```python
from build123d import *

# Parameters (mm, degrees)
BOSS_EXTRUDE1_DEPTH = 50
SHELL1_T            = -1.5
SKETCH2_R           = 2.5
CUT_EXTRUDE1_DEPTH  = 50
SKETCH3_OUTSIDE_W   = 189.504
SKETCH3_OUTSIDE_H   = 139.504
CUT_EXTRUDE2_DEPTH  = 5
CUT_EXTRUDE2_TAPER  = 0.5
FILLET1_R           = 0.5
CHAMFER1_SIZE       = 1.25


with BuildPart() as part:
    # Sketch1 → Boss-Extrude1 (new body)
    with BuildSketch(Plane(origin=(0, 0, 0), x_dir=(1, 0, 0), z_dir=(0, 1, 0))):
        with BuildLine():
            Line((-72.5, -50), (72.5, -50))
            ThreePointArc((72.5, -50), (74.267766953, -49.267766953), (75, -47.5))
            Line((75, -47.5), (75, 47.5))
            ThreePointArc((75, 47.5), (74.267766953, 49.267766953), (72.5, 50))
            Line((72.5, 50), (-72.5, 50))
            ThreePointArc((-72.5, 50), (-74.267766953, 49.267766953), (-75, 47.5))
            Line((-75, 47.5), (-75, -47.5))
            ThreePointArc((-75, -47.5), (-74.267766953, -49.267766953), (-72.5, -50))
        make_face()
    extrude(amount=BOSS_EXTRUDE1_DEPTH)

    # Shell1
    shell1_openings = [part.faces().sort_by_distance(p)[0] for p in [
        (0, 50, 0),
    ]]
    offset(amount=SHELL1_T, openings=shell1_openings, kind=Kind.INTERSECTION)

    # Sketch2 → Cut-Extrude1 (cut)
    with BuildSketch(Plane(origin=(0, 1.5, 0), x_dir=(1, 0, 0), z_dir=(0, 1, 0))):
        with Locations((-65, 40)):
            Circle(SKETCH2_R)
        with Locations((65, 40)):
            Circle(SKETCH2_R)
        with Locations((65, -40)):
            Circle(SKETCH2_R)
        with Locations((-65, -40)):
            Circle(SKETCH2_R)
    extrude(amount=-CUT_EXTRUDE1_DEPTH, mode=Mode.SUBTRACT)

    # Sketch3 outside → Cut-Extrude2 (cut)
    with BuildSketch(Plane(origin=(0, 50, 0), x_dir=(1, 0, 0), z_dir=(0, 1, 0))):
        Rectangle(SKETCH3_OUTSIDE_W, SKETCH3_OUTSIDE_H)
        with BuildLine():
            Line((-69.232233047, -45.732233047), (69.232233047, -45.732233047))
            ThreePointArc((69.232233047, -45.732233047), (70.292893219, -45.292893219), (70.732233047, -44.232233047))
            Line((70.732233047, -44.232233047), (70.732233047, 44.232233047))
            ThreePointArc((70.732233047, 44.232233047), (70.292893219, 45.292893219), (69.232233047, 45.732233047))
            Line((69.232233047, 45.732233047), (-69.232233047, 45.732233047))
            ThreePointArc((-69.232233047, 45.732233047), (-70.292893219, 45.292893219), (-70.732233047, 44.232233047))
            Line((-70.732233047, 44.232233047), (-70.732233047, -44.232233047))
            ThreePointArc((-70.732233047, -44.232233047), (-70.292893219, -45.292893219), (-69.232233047, -45.732233047))
        make_face(mode=Mode.SUBTRACT)
    extrude(amount=-CUT_EXTRUDE2_DEPTH, taper=CUT_EXTRUDE2_TAPER, mode=Mode.SUBTRACT)

    # Fillet1
    fillet1_edges = [part.edges().sort_by_distance(p)[0] for p in [
        (-75, 0, 0),
        (-74.267766953, 0, -49.267766953),
        (0, 0, -50),
        (74.267766953, 0, -49.267766953),
        (75, 0, 0),
        (74.267766953, 0, 49.267766953),
        (0, 0, 50),
        (-74.267766953, 0, 49.267766953),
    ]]
    fillet(fillet1_edges, radius=FILLET1_R)

    # Chamfer1
    chamfer1_edges = [part.edges().sort_by_distance(p)[0] for p in [
        (-67.5, 1.5, -40),
        (62.5, 1.5, -40),
        (62.5, 1.5, 40),
        (-67.5, 1.5, 40),
    ]]
    chamfer(chamfer1_edges, length=CHAMFER1_SIZE)


solid = part.part
```
CAD build for the part. Positions are in the model's coordinates, mm. A direction names the side the tool comes from. Coordinates: 2 decimals unless noted, no trailing zeros. Order: outer loops, then holes, each group sorted by start corner. A loop starts at its lowest first (then second) coordinate and runs counter-clockwise, first axis right, second up. Notation, with made-up numbers: (-36.5, 78) -> (-6.5, 78) arc R12 cw to (-6.5, 83) -> close; hole circle Ø7 at (71, -37). An arc over 180 degrees is marked (long way). Use one line per item in the form item = value. Start each with the question number.
1) Drill centre lines: L1, parallel to Z at x = 65.5, y = 11.5; L2, parallel to X at y = 15.5, z = -34.5; L3, parallel to X at y = 0.1, z = 40. Where is each one in solid material? Low to high. Write a range as [from, to].
2) Band-saw the part on A-A on z = -40. Give the cut face in (x, y), then the cut area to 3 significant figures.
3) Band-saw the part on B-B on x = -65. Give the cut face in (y, z), then the cut area to 3 significant figures.
4) Drop flat-ended pins along their axis: pin 1 (2 mm diameter, centred on x = -42, z = -29.5, fed in from +Y); pin 2 (4.5 mm diameter, centred on x = 65, z = 40, fed in from -Y); pin 3 (6 mm diameter, centred on x = -65, z = 40, fed in from +Y). Give the stop position or say it passes through.
5) Band-saw the part on C-C on y = 32. Give the cut face in (x, z), then the cut area to 3 significant figures.
6) Band-saw the part on D-D on z = 29. Give the cut face in (x, y).
7) Tool access for faces 1 (the flat face through (1, 23, -48.5)), 2 (the flat face through (-1, 22, 50)): list every direction of +Z, -Z, +X, -X, +Y, -Y with a clear straight run to the whole face (end or side of a thin tool).
8) Pull direction X, two halves, no side cores. Call faces 3 (the flat face through (-1, 1.5, -1)), 4 (the flat face through (-14, 45, 49)), 5 (the flat face through (75, 22, 1)): +X half, -X half, draft (parallel to the pull), parting line (faces both ways), or undercut.
Entries:
q1.L1 = [-50, -48.5], [48.5, 50]
q1.L2 = [-75, -73.5], [73.5, 75]
q1.L3 = [-74.8, -67.5], [-62.5, 62.5], [67.5, 74.8]
q2.outline = (-75, 0.5) arc R0.5 ccw to (-74.5, 0) -> (-67.5, 0) -> (-67.5, 0.25) -> (-68.75, 1.5) -> (-73.5, 1.5) -> (-73.5, 45) -> (-75, 45) -> close; (-62.5, 0) -> (62.5, 0) -> (62.5, 0.25) -> (61.25, 1.5) -> (-61.25, 1.5) -> (-62.5, 0.25) -> close; (67.5, 0) -> (74.5, 0) arc R0.5 ccw to (75, 0.5) -> (75, 45) -> (73.5, 45) -> (73.5, 1.5) -> (68.75, 1.5) -> (67.5, 0.25) -> close
q2.area = 337 mm2
q3.outline = (0, -49.5) arc R0.5 ccw to (0.5, -50) -> (45, -50) -> (45, -48.5) -> (1.5, -48.5) -> (1.5, -43.75) -> (0.25, -42.5) -> (0, -42.5) -> close; (0, -37.5) -> (0.25, -37.5) -> (1.5, -36.25) -> (1.5, 36.25) -> (0.25, 37.5) -> (0, 37.5) -> close; (0, 42.5) -> (0.25, 42.5) -> (1.5, 43.75) -> (1.5, 48.5) -> (45, 48.5) -> (45, 50) -> (0.5, 50) arc R0.5 ccw to (0, 49.5) -> close
q3.area = 262 mm2
q4.pin_1 = 1.5
q4.pin_2 = through
q4.pin_3 = 0.75
q5.outline = (-75, -47.5) arc R2.5 ccw to (-72.5, -50) -> (72.5, -50) arc R2.5 ccw to (75, -47.5) -> (75, 47.5) arc R2.5 ccw to (72.5, 50) -> (-72.5, 50) arc R2.5 ccw to (-75, 47.5) -> close; hole (-73.5, -47.5) arc R1 ccw to (-72.5, -48.5) -> (72.5, -48.5) arc R1 ccw to (73.5, -47.5) -> (73.5, 47.5) arc R1 ccw to (72.5, 48.5) -> (-72.5, 48.5) arc R1 ccw to (-73.5, 47.5) -> close
q5.area = 736 mm2
q6.outline = (-75, 0.5) arc R0.5 ccw to (-74.5, 0) -> (74.5, 0) arc R0.5 ccw to (75, 0.5) -> (75, 45) -> (73.5, 45) -> (73.5, 1.5) -> (-73.5, 1.5) -> (-73.5, 45) -> (-75, 45) -> close
q7.face_1 = +Y
q7.face_2 = +Z, +X, -X, +Y, -Y
q8.face_3 = undercut
q8.face_4 = draft
q8.face_5 = +X half
